Geometry: final body of the model. Coordinates: model frame, mm. Face numbers are marked on the shaded views. Give positions to 0.01 mm unless a question says otherwise; leave off trailing zeros. Loops run counter-clockwise (first coordinate to the right, second up) from the corner with the lowest first, then second, coordinate; pieces in that order, holes last.
1. Section C-C, the plane x = 56. Output: boundary loops of the cut face in (y, z).
2. Material intervals for line 1 along Y through (x, z) = (0, 4); line 2 along Z through (x, y) = (-30, -72); line 3 along Y through (x, z) = (0, 28.6), sorted ascending.
3. First-contact query: P1, Ø5.5, axis at x = -39, z = 13.5, coming from the +Y side; P2, Ø4, axis at x = -42, z = 13.5, coming from the -Y side; P3, Ø4, axis at y = 14, z = 9, coming from the +X side. Flat tips, straight axial feed; report the tip coordinate or a pass-through.
4. Section B-B, the plane y = 25. Output: boundary loops of the cut face in (x, z).
5. Section A-A, the plane x = 0. Output: boundary loops of the cut face in (y, z), then the cut area to 4 significant figures.
6. Draft query along Y for the marked faces 1, 2, 3 and 4. Return one class per face: +Y half, -Y half, draft (parallel to the pull), parting line (faces both ways), or undercut.
7. Section D-D, the plane z = 20.75. Output: boundary loops of the cut face in (x, y).
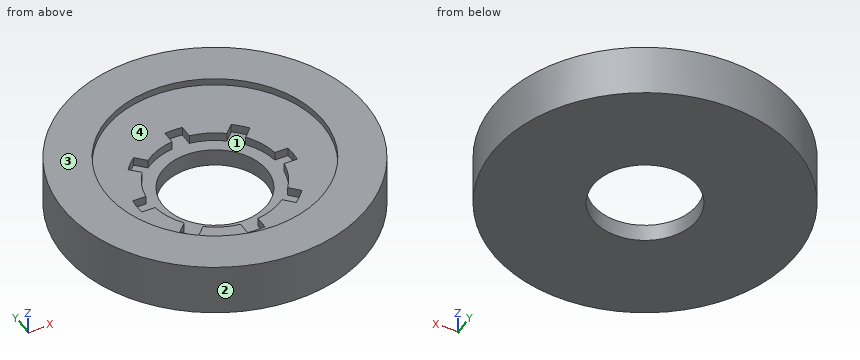
from build123d import *

# Parameters (mm, degrees)
F0_R     = 87.5
F0_R_2   = 30
F1_DEPTH = 10
F2_R     = 87.5
F2_R_2   = 37.5
F3_DEPTH = 5
F5_DEPTH = 5
F6_R     = 87.5
F6_R_2   = 62.5
F7_DEPTH = 15
F8_R     = 77.5
F9_DEPTH = 11


with BuildPart() as f1:
    # F0 (on Top) → F1 (new body)
    with BuildSketch(Plane.XY):
        Circle(F0_R)
        Circle(F0_R_2, mode=Mode.SUBTRACT)
    extrude(amount=F1_DEPTH)

    # F2 (on face) → F3 (join)
    with BuildSketch(Plane.XY.offset(10)):
        Circle(F2_R)
        Circle(F2_R_2, mode=Mode.SUBTRACT)
    extrude(amount=F3_DEPTH)

    # F4 (on face) → F5 (cut)
    with BuildSketch(Plane.XY.offset(15)):
        with BuildLine():
            ThreePointArc((-29.815278958, 22.7442111461), (-26.5165042945, 26.5165042945), (-22.7442111461, 29.815278958))
            Line((-22.7442111461, 29.815278958), (-28.0872426958, 35.1583105076))
            ThreePointArc((-28.0872426958, 35.1583105076), (-31.8198051534, 31.8198051534), (-35.1583105076, 28.0872426958))
            Line((-35.1583105076, 28.0872426958), (-29.815278958, 22.7442111461))
        make_face()
        with BuildLine():
            Line((-5, 44.72135955), (-5, 37.1651718683))
            ThreePointArc((-5, 37.1651718683), (0, 37.5), (5, 37.1651718683))
            Line((5, 37.1651718683), (5, 44.72135955))
            ThreePointArc((5, 44.72135955), (0, 45), (-5, 44.72135955))
        make_face()
        with BuildLine():
            Line((28.0872426958, 35.1583105076), (22.7442111461, 29.815278958))
            ThreePointArc((22.7442111461, 29.815278958), (26.5165042945, 26.5165042945), (29.815278958, 22.7442111461))
            Line((29.815278958, 22.7442111461), (35.1583105076, 28.0872426958))
            ThreePointArc((35.1583105076, 28.0872426958), (31.8198051534, 31.8198051534), (28.0872426958, 35.1583105076))
        make_face()
        with BuildLine():
            Line((44.72135955, 5), (37.1651718683, 5))
            ThreePointArc((37.1651718683, 5), (37.4161993331, 2.5055992236), (37.5, 0))
            ThreePointArc((37.5, 0), (37.4161993331, -2.5055992236), (37.1651718683, -5))
            Line((37.1651718683, -5), (44.72135955, -5))
            ThreePointArc((44.72135955, -5), (44.9302858869, -2.5038790157), (45, 0))
            ThreePointArc((45, 0), (44.9302858869, 2.5038790157), (44.72135955, 5))
        make_face()
        with BuildLine():
            Line((35.1583105076, -28.0872426958), (29.815278958, -22.7442111461))
            ThreePointArc((29.815278958, -22.7442111461), (26.5165042945, -26.5165042945), (22.7442111461, -29.815278958))
            Line((22.7442111461, -29.815278958), (28.0872426958, -35.1583105076))
            ThreePointArc((28.0872426958, -35.1583105076), (31.8198051534, -31.8198051534), (35.1583105076, -28.0872426958))
        make_face()
        with BuildLine():
            ThreePointArc((5, -37.1651718683), (0, -37.5), (-5, -37.1651718683))
            Line((-5, -37.1651718683), (-5, -44.72135955))
            ThreePointArc((-5, -44.72135955), (0, -45), (5, -44.72135955))
            Line((5, -44.72135955), (5, -37.1651718683))
        make_face()
        with BuildLine():
            ThreePointArc((-22.7442111461, -29.815278958), (-26.5165042945, -26.5165042945), (-29.815278958, -22.7442111461))
            Line((-29.815278958, -22.7442111461), (-35.1583105076, -28.0872426958))
            ThreePointArc((-35.1583105076, -28.0872426958), (-31.8198051534, -31.8198051534), (-28.0872426958, -35.1583105076))
            Line((-28.0872426958, -35.1583105076), (-22.7442111461, -29.815278958))
        make_face()
        with BuildLine():
            ThreePointArc((-37.1651718683, -5), (-37.5, 0), (-37.1651718683, 5))
            Line((-37.1651718683, 5), (-44.72135955, 5))
            ThreePointArc((-44.72135955, 5), (-45, 0), (-44.72135955, -5))
            Line((-44.72135955, -5), (-37.1651718683, -5))
        make_face()
    extrude(amount=-F5_DEPTH, mode=Mode.SUBTRACT)

    # F6 (on face) → F7 (join)
    with BuildSketch(Plane.XY.offset(15)):
        Circle(F6_R)
        Circle(F6_R_2, mode=Mode.SUBTRACT)
    extrude(amount=F7_DEPTH)

    # F8 (on face) → F9 (cut)
    with BuildSketch(Plane.XY.offset(15)):
        with Locations((0, -1.9303644706)):
            Circle(F8_R)
    extrude(amount=F9_DEPTH, mode=Mode.SUBTRACT)


solid = f1.part
Answers below:
1. outline: (-67.23, 0) - (67.23, 0) - (67.23, 30) - (27.75, 30) - (27.75, 26) - (51.64, 26) - (51.64, 15) - (-55.51, 15) - (-55.51, 26) - (-27.75, 26) - (-27.75, 30) - (-67.23, 30) - close
2. line 1: y = -87.5 to -30, 30 to 87.5
2. line 2: z = 0 to 15, 26 to 30
2. line 3: y = -87.5 to -62.5, 62.5 to 87.5
3. P1: stops at y = 79.64
3. P2: stops at y = -77.82
3. P3: stops at x = 86.67
4. outline: (-83.85, 0) - (-16.58, 0) - (-16.58, 10) - (-32.07, 10) - (-32.07, 15) - (-72.67, 15) - (-72.67, 26) - (-57.28, 26) - (-57.28, 30) - (-83.85, 30) - close; (16.58, 0) - (83.85, 0) - (83.85, 30) - (57.28, 30) - (57.28, 26) - (72.67, 26) - (72.67, 15) - (32.07, 15) - (32.07, 10) - (16.58, 10) - close
5. outline: (-87.5, 0) - (-30, 0) - (-30, 10) - (-45, 10) - (-45, 15) - (-79.43, 15) - (-79.43, 26) - (-62.5, 26) - (-62.5, 30) - (-87.5, 30) - close; (30, 0) - (87.5, 0) - (87.5, 30) - (62.5, 30) - (62.5, 26) - (75.57, 26) - (75.57, 15) - (45, 15) - (45, 10) - (30, 10) - close
5. area: 1,995 mm2
6. face 1: undercut
6. face 2: parting line
6. face 3: draft
6. face 4: undercut
7. outline: circle Ø175 at (0, 0); hole circle Ø155 at (0, -1.93)
